Geometry check sheet. Reference: drawing and pictorial views, mm from the part's lowest x, y, z. A direction names the side the tool comes from. Give positions to 0.01 mm unless a question says otherwise; leave off trailing zeros. Order: outer loops, then holes, each group sorted by start corner. A loop starts at its lowest first (then second) coordinate and runs counter-clockwise, first axis right, second up.
Item 1: Release check for a two-part mould opening along X. For the marked faces 3, 4 and 5 record: released by +X, released by -X, zero draft, split by the parting line, or undercut.
Item 2: Sectioned sample at D-D on z = 2.5. Record the boundary of the cut face in (x, y).
Item 3: Sectioned sample at A-A on y = 18. Record the boundary of the cut face in (x, z).
Item 4: Gauge pin test, flat end, axial feed: P1, Ø4, axis at y = 11.5, z = 3, coming from the +X side. Record the tip position at first contact, or that the pin passes through.
Item 5: Access from +Z, -Z, +X, -X, +Y, -Y to the whole of each face (thin tool, end or side, straight path). Record for the marked faces 1 and 2.
Item 6: Sectioned sample at C-C on z = 4. Record the boundary of the cut face in (x, y), and give its area (3 significant figures).
Item 7: Material ranges on line 1 along Z through (x, y) = (18, 3); line 2 along X through (y, z) = (9.75, 7.5), recorded low to high.
Item 8: Sectioned sample at B-B on x = 17.75. Record the boundary of the cut face in (y, z).
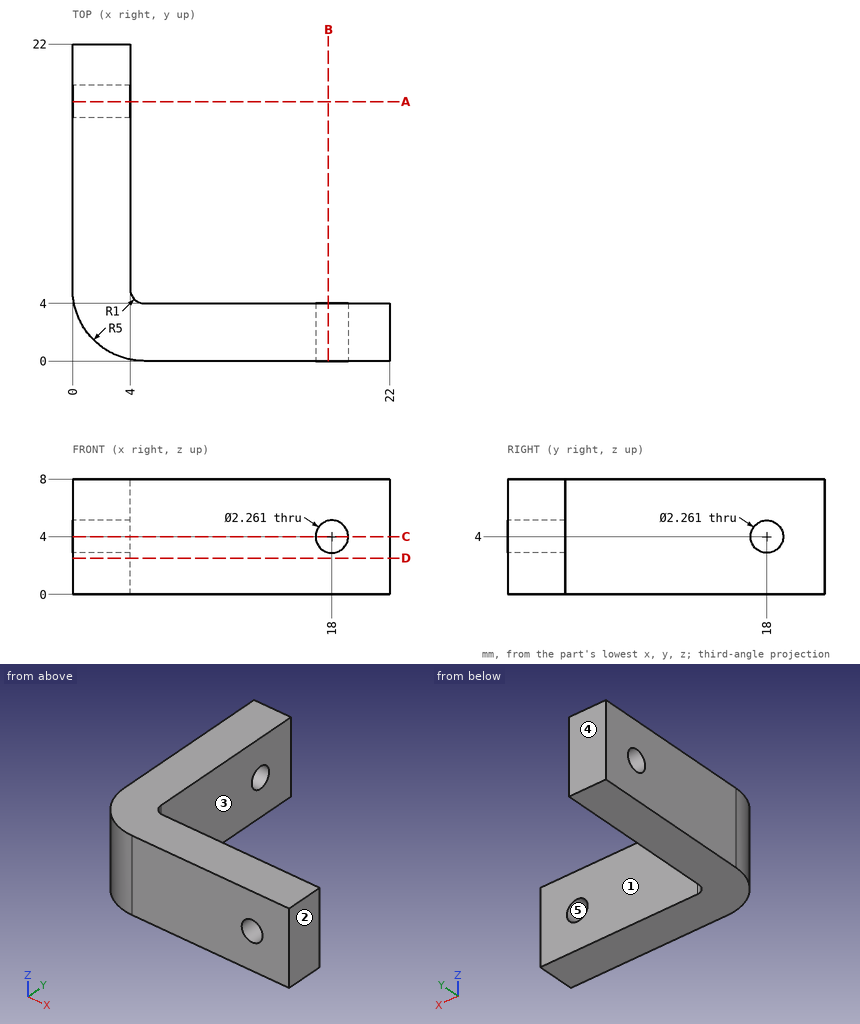
Report:
1. face 3: released by +X
1. face 4: zero draft
1. face 5: undercut
2. outline: (0, 5) arc R5 ccw to (5, 0) - (22, 0) - (22, 4) - (5, 4) arc R1 cw to (4, 5) - (4, 22) - (0, 22) - close
3. outline: (0, 0) - (4, 0) - (4, 2.87) - (0, 2.87) - close; (0, 5.13) - (4, 5.13) - (4, 8) - (0, 8) - close
4. P1: stops at x = 4
5. face 1: +Z, -Z, +X, +Y
5. face 2: +Z, -Z, +X, +Y, -Y
6. outline: (0, 5) arc R5 ccw to (5, 0) - (16.87, 0) - (16.87, 4) - (5, 4) arc R1 cw to (4, 5) - (4, 16.87) - (0, 16.87) - close; (0, 19.13) - (4, 19.13) - (4, 22) - (0, 22) - close; (19.13, 0) - (22, 0) - (22, 4) - (19.13, 4) - close
6. area: 137 mm2
7. line 1: z = 0 to 2.87, 5.13 to 8
7. line 2: x = 0 to 4
8. outline: (0, 0) - (4, 0) - (4, 2.9) - (0, 2.9) - close; (0, 5.1) - (4, 5.1) - (4, 8) - (0, 8) - close
